CAD build for the part. Positions are in the model's coordinates, mm. A direction names the side the tool comes from. Give positions to 0.01 mm unless a question says otherwise; leave off trailing zeros. Loops run counter-clockwise (first coordinate to the right, second up) from the corner with the lowest first, then second, coordinate; pieces in that order, holes last.
Item 1: Mould opens along Y. For faces 4 (the flat face through (6, 4, 5)), 5 (the flat face through (0.5, 1.5, 5)), 6 (the flat face through (9, 7.5, 1)) say: released by +Y, released by -Y, zero draft, split by the parting line, or undercut.
Item 2: Saw through at B-B on y = 6. Give the cut face in (x, z).
Item 3: Probe probe 1 along Z at (x, y) = (5, 1.9); probe 2 along X at (y, z) = (1.75, 8); probe 3 along Z at (x, y) = (5, 2.2). List the from-to ranges inside material, lowest first.
Item 4: Saw through at C-C on x = 7.5. Give the cut face in (y, z), plus the area to 3 significant figures.
Item 5: Saw through at D-D on y = 2.25. Give the cut face in (x, z), plus the area to 3 significant figures.
Item 6: Which spindle directions (+Z, -Z, +X, -X, +Y, -Y) get a long thin tool onto all of the face, cutting with end or side? Do faces 1 (the flat face through (3, 3.5, 5)), 2 (the flat face through (4.5, 7, 2.5)), 3 (the flat face through (1, 5, 1)). Say none if no direction does.
Item 7: Saw through at A-A on z = 1.5. Give the cut face in (x, y).
Item 8: Drop flat-ended pins along their axis: P1, Ø1.5, axis at x = 7.5, y = 5.5, coming from the +Z side; P2, Ø3, axis at x = 3.5, z = 3, coming from the -Y side; P3, Ø2.5, axis at x = 4, z = 10.5, coming from the +Y side; P4, Ø4.5, axis at x = 7.5, y = 10, coming from the +Z side. Give the stop position or say it passes through.
from build123d import *

# Parameters (mm, degrees)
BOSS_EXTRUDE1_DEPTH = 1
BOSS_EXTRUDE3_DEPTH = 2
SKETCH5_W           = 6.323405325
SKETCH5_H           = 4.405706714
CUT_EXTRUDE2_DEPTH  = 1
SKETCH6_W           = 9
SKETCH6_H           = 4
BOSS_EXTRUDE4_DEPTH = 2
SKETCH7_W           = 10
SKETCH7_H           = 3
BOSS_EXTRUDE5_DEPTH = 8
SKETCH8_R           = 3
CUT_EXTRUDE3_DEPTH  = 8
CUT_EXTRUDE4_DEPTH  = 1
CUT_EXTRUDE5_DEPTH  = 1
BOSS_EXTRUDE6_DEPTH = 1


with BuildPart() as part:
    # Sketch2 → Boss-Extrude1 (new body)
    with BuildSketch(Plane.XY):
        with BuildLine():
            Line((0, 0), (0, 4))
            Line((0, 4), (4.649234196, 9.863840158))
            ThreePointArc((4.649234196, 9.863840158), (7.986839041, 10.833045836), (10, 8))
            Line((10, 8), (10, 0))
            Line((10, 0), (0, 0))
        make_face()
        with BuildLine():
            Line((9, 8), (9, 7))
            ThreePointArc((9, 7), (7, 5), (5, 7))
            Line((5, 7), (5, 8))
            ThreePointArc((5, 8), (7, 10), (9, 8))
        make_face(mode=Mode.SUBTRACT)
    extrude(amount=BOSS_EXTRUDE1_DEPTH)

    # Sketch3 → Boss-Extrude3 (add)
    with BuildSketch(Plane.XY.offset(1)):
        with BuildLine():
            Line((1, 4), (1, 0))
            Line((1, 0), (10, 0))
            Line((10, 0), (10, 8))
            ThreePointArc((10, 8), (7, 11), (4, 8))
            Line((4, 8), (4, 7))
            Line((4, 7), (1, 4))
        make_face()
        with BuildLine():
            Line((5, 7), (5, 8))
            ThreePointArc((5, 8), (7, 10), (9, 8))
            Line((9, 8), (9, 7))
            ThreePointArc((9, 7), (7, 5), (5, 7))
        make_face(mode=Mode.SUBTRACT)
    extrude(amount=BOSS_EXTRUDE3_DEPTH)

    # Sketch5 → Cut-Extrude2 (cut)
    with BuildSketch(Plane.XY.offset(3)):
        with Locations((7.161702663, 9.202853357)):
            Rectangle(SKETCH5_W, SKETCH5_H)
    extrude(amount=-CUT_EXTRUDE2_DEPTH, mode=Mode.SUBTRACT)

    # Sketch6 → Boss-Extrude4 (add)
    with BuildSketch(Plane.XY.offset(3)):
        with Locations((5.5, 2)):
            Rectangle(SKETCH6_W, SKETCH6_H)
    extrude(amount=BOSS_EXTRUDE4_DEPTH)

    # Sketch7 → Boss-Extrude5 (add)
    with BuildSketch(Plane.XY.offset(5)):
        with Locations((5, 1.5)):
            Rectangle(SKETCH7_W, SKETCH7_H)
    extrude(amount=BOSS_EXTRUDE5_DEPTH)

    # Sketch8 → Cut-Extrude3 (cut)
    with BuildSketch(Plane(origin=(0, 4, 0), x_dir=(1, 0, 0), z_dir=(0, 1, 0))):
        with BuildLine():
            Line((10, -16.316770955), (10, -8))
            ThreePointArc((10, -8), (5, -13), (0, -8))
            Line((0, -8), (0, -16.316770955))
            Line((0, -16.316770955), (10, -16.316770955))
        make_face()
        with Locations((5, -8)):
            Circle(SKETCH8_R)
    extrude(amount=-CUT_EXTRUDE3_DEPTH, mode=Mode.SUBTRACT)

    # Sketch9 → Cut-Extrude4 (cut)
    with BuildSketch(Plane.XZ):
        with BuildLine():
            Line((5, 11), (5, 13))
            ThreePointArc((5, 13), (1.464466094, 11.535533906), (0, 8))
            Line((0, 8), (2, 8))
            ThreePointArc((2, 8), (2.878679656, 10.121320344), (5, 11))
        make_face()
    extrude(amount=-CUT_EXTRUDE4_DEPTH, mode=Mode.SUBTRACT)

    # Sketch10 → Cut-Extrude5 (cut)
    with BuildSketch(Plane(origin=(0, 3, 0), x_dir=(1, 0, 0), z_dir=(0, 1, 0))):
        with BuildLine():
            Line((0, -8), (2, -8))
            ThreePointArc((2, -8), (5, -11), (8, -8))
            Line((8, -8), (10, -8))
            ThreePointArc((10, -8), (5, -13), (0, -8))
        make_face()
    extrude(amount=-CUT_EXTRUDE5_DEPTH, mode=Mode.SUBTRACT)

    # Sketch11 → Boss-Extrude6 (add)
    with BuildSketch(Plane(origin=(0, 3, 0), x_dir=(1, 0, 0), z_dir=(0, 1, 0))):
        with BuildLine():
            Line((8, -8), (10, -8))
            Line((10, -8), (10, -5))
            Line((10, -5), (5, -5))
            ThreePointArc((5, -5), (7.121320344, -5.878679656), (8, -8))
        make_face()
    extrude(amount=BOSS_EXTRUDE6_DEPTH)


solid = part.part
Results below:
1. face 4: released by +Y
1. face 5: zero draft
1. face 6: undercut
2. outline: (1.59, 0) - (5.27, 0) - (5.27, 3) - (3, 3) - (3, 1) - (1.59, 1) - close; (8.73, 0) - (10, 0) - (10, 3) - (8.73, 3) - close
3. probe 1: z = 0 to 5, 11 to 13
3. probe 2: x = 0 to 2, 8 to 10
3. probe 3: z = 0 to 5
4. outline: (0, 0) - (5.06, 0) - (5.06, 3) - (4, 3) - (4, 6.34) - (0, 6.34) - close; (0, 9.66) - (2, 9.66) - (2, 12.33) - (0, 12.33) - close; (9.94, 0) - (10.96, 0) - (10.96, 2) - (9.94, 2) - close
4. area: 35.9 mm2
5. outline: (0, 0) - (10, 0) - (10, 8) - (8, 8) arc R3 cw to (2, 8) - (0, 8) - (0, 5) - (1, 5) - (1, 1) - (0, 1) - close
5. area: 61.9 mm2
6. face 1: +Z, -X, +Y
6. face 2: +Z, +X, -X, +Y
6. face 3: -X, +Y
7. outline: (1, 0) - (10, 0) - (10, 8) arc R3 ccw to (4, 8) - (4, 7) - (1, 4) - close; hole (5, 7) arc R2 ccw to (9, 7) - (9, 8) arc R2 ccw to (5, 8) - close
8. P1: stops at z = 3
8. P2: stops at y = 0
8. P3: stops at y = 2
8. P4: stops at z = 2
